from build123d import *

# Parameters (mm, degrees)
SKETCH_1_W             = 137
SKETCH_1_H             = 30
EXTRUDE_1_DEPTH        = 10
HOLE_WIZARD_M5_1_D     = 5.5
EXTRUDE_2_DEPTH        = 20
PATTERN_LINEAR_1_COUNT = 8
PATTERN_LINEAR_1_PITCH = 15
EXTRUDE_4_DEPTH        = 20


with BuildPart() as part:
    # 草图1 → 凸台-拉伸1 (new, symmetric)
    with BuildSketch(Plane(origin=(0, 0, 0), x_dir=(0, 0, -1), z_dir=(1, 0, 0))):
        Rectangle(SKETCH_1_W, SKETCH_1_H)
    extrude(amount=EXTRUDE_1_DEPTH, both=True)

    # M5 间隙孔1 (through all)
    with Locations(Plane(origin=(10, 0, 0), x_dir=(0, 0, -1), z_dir=(1, 0, 0))):
        with Locations((-63.5, -10), (63.5, -10)):
            Hole(HOLE_WIZARD_M5_1_D / 2)

    # 草图4 → 凸台-拉伸2 (add)
    with BuildSketch(Plane(origin=(0, 15, 0), x_dir=(1, 0, 0), z_dir=(0, 1, 0))):
        Polygon((6.92820323, -52.5), (3.464101615, -46.5), (-3.464101615, -46.5), (-6.92820323, -52.5), (-3.464101615, -58.5), (3.464101615, -58.5), align=None)
    extrude_2 = extrude(amount=EXTRUDE_2_DEPTH)

    # 草图6 → 旋转1 (revolve)
    with BuildSketch(Plane(origin=(0, 0, 0), x_dir=(0, 0, -1), z_dir=(1, 0, 0)), mode=Mode.PRIVATE) as revolve_1_sk:
        Polygon((-52.5, -15), (-49.5, -15), (-49.5, -20), (-47.5, -20), (-47.5, -25), (-52.5, -25), align=None)
    revolve_1 = revolve(revolve_1_sk.sketch.rotate(Axis((0, 35, 52.5), (0, -1, 0)), 180), axis=Axis((0, 35, 52.5), (0, -1, 0)))

    # 阵列(线性)1: 凸台-拉伸2, 旋转1 ×8
    with Locations(*[(0, 0, -i * PATTERN_LINEAR_1_PITCH) for i in range(1, PATTERN_LINEAR_1_COUNT)]):
        add(extrude_2)
        add(revolve_1)

    # 草图5 → 凸台-拉伸4 (add)
    with BuildSketch(Plane.XY.offset(68.5)):
        Polygon((3.464101615, 6), (-3.464101615, 6), (-6.92820323, 0), (-3.464101615, -6), (3.464101615, -6), (6.92820323, 0), align=None)
    extrude(amount=EXTRUDE_4_DEPTH)


solid = part.part
Geometry check sheet. Reference: the model listing, model coordinates, mm. A direction names the side the tool comes from. Coordinates: 2 decimals unless noted, no trailing zeros. Write each loop counter-clockwise with the first axis right and the second up, starting at its lowest first coordinate (ties: lowest second). Pieces come first, ordered by that corner, then holes. Notation, with made-up numbers: (-21, 89) -> (-12, 89) arc R25 cw to (-12, 112) -> close; hole circle Ø1 at (40, 56). An arc over 180 degrees is marked (long way). One line per question, with ' | ' between items.
1. Set-up check for faces 1 (the flat face through (0, 25, 28.5)), 2 (the flat face through (0, 25, 58.5)), 3 (the cylindrical face through (-0.22, -22.535, -27.495)), 4 (the flat face through (-5.22, 24.86, 10.46)): record each of +Z, -Z, +X, -X, +Y, -Y from which the full face is reachable in a straight line by a thin tool's end or side.
Answers:
face 1: +X, -X, +Y | face 2: +Z, +X, -X, +Y | face 3: -Y | face 4: -X, +Y
2. Cross-section at C-C on y = -4. Record the cut outline in (x, z).
Answers:
outline: (-10, -68.5) -> (10, -68.5) -> (10, 68.5) -> (4.62, 68.5) -> (4.62, 88.5) -> (-4.62, 88.5) -> (-4.62, 68.5) -> (-10, 68.5) -> close
3. Depth check by flat-ended pin: pin 1 Ø5.5 at (x, y) = (-1, 28) entering from -Z; pin 2 Ø3.5 at (x, y) = (0.5, 26) entering from +Z; pin 3 Ø2 at (x, z) = (-1.5, 83) entering from +Y. Enter the tip coordinate at first touch or a pass-through.
Answers:
pin 1: stops at z = -58.5 | pin 2: stops at z = 58.5 | pin 3: stops at y = 6
4. Cross-section at B-B on z = 63.5. Record the cut outline in (x, y).
Answers:
outline: (-10, -15) -> (10, -15) -> (10, -12.75) -> (-10, -12.75) -> close; (-10, -7.25) -> (10, -7.25) -> (10, 15) -> (-10, 15) -> close
5. Draft check along Y on faces 5 (the flat face through (-5.172, 24.86, -40.542)), 6 (the flat face through (2, -20, 5)), 7 (the flat face through (2, -20, 20)), 8 (the flat face through (0, -6, 78)). Enter one of: +Y half, -Y half, draft (parallel to the pull), parting line (faces both ways), or undercut.
Answers:
face 5: draft | face 6: undercut | face 7: undercut | face 8: -Y half
6. Thickness scan on probe 1 along Y at (x, z) = (3.25, -63.5); probe 2 along Z at (x, y) = (4.25, -7.5); probe 3 along Y at (x, z) = (-1, 45.5). Record the ranges inside material, lowest first. Write a range as from..to.
Answers:
probe 1: y = -15..-12.75, -7.25..15 | probe 2: z = -68.5..-64.65, -62.35..62.35, 64.65..68.5 | probe 3: y = -15..15
7. Cross-section at A-A on y = -10. Record the cut outline in (x, z).
Answers:
outline: (-10, -68.5) -> (10, -68.5) -> (10, -66.25) -> (-10, -66.25) -> close; (-10, -60.75) -> (10, -60.75) -> (10, 60.75) -> (-10, 60.75) -> close; (-10, 66.25) -> (10, 66.25) -> (10, 68.5) -> (-10, 68.5) -> close
8. Cross-section at D-D on z = -51. Record the cut outline in (x, y).
Answers:
outline: (-10, -15) -> (-2.6, -15) -> (-2.6, -20) -> (-4.77, -20) -> (-4.77, -25) -> (4.77, -25) -> (4.77, -20) -> (2.6, -20) -> (2.6, -15) -> (10, -15) -> (10, 15) -> (6.06, 15) -> (6.06, 35) -> (-6.06, 35) -> (-6.06, 15) -> (-10, 15) -> close
